Check sheet for the modelled part. Datum: model origin and axes. Units: mm. Face numbers are marked on the shaded views. Give positions to 0.01 mm unless a question says otherwise; leave off trailing zeros. Order: outer loops, then holes, each group sorted by start corner. A loop starts at its lowest first (then second) coordinate and runs counter-clockwise, first axis right, second up. Notation, with made-up numbers: (-1.5, 73) -> (2.5, 73) arc R15 cw to (2.5, 98) -> close; hole circle Ø10 at (80.25, 60.25). An arc over 180 degrees is marked (long way). Answer in a Markdown table with one row per item. Add a question column.
(1) Cross-section at D-D (y = 5). Record the cut outline in (x, z), then the cut area to 3 significant figures.
(2) Cross-section at A-A (z = 9.25). Record the cut outline in (x, y).
(3) Thickness scan on L1, parallel to Y at x = 15, z = 1.5; L2, parallel to X at y = 6, z = 7.75; L3, parallel to Y at x = -6.2, z = 13.25. Record the ranges inside material, lowest first. Write a range as [from, to].
(4) Release check for a two-part mould opening along X. For the marked faces 1, 2, 3 and 4 record: released by +X, released by -X, zero draft, split by the parting line, or undercut.
(5) Cross-section at C-C (z = 5.75). Record the cut outline in (x, y), then the cut area to 3 significant figures.
(6) Go/stop test with flat-tipped pins: pin 1 (1 mm diameter, centred on x = -11, y = 2, fed in from +Z); pin 2 (4.5 mm diameter, centred on y = -7.5, z = 5.75, fed in from +X); pin 3 (4.5 mm diameter, centred on y = 4, z = 10, fed in from -X); pin 4 (1.5 mm diameter, centred on x = 9, z = 5.5, fed in from -Y). Record where each tip stops, or that it passes through.
(7) Cross-section at B-B (x = 15). Record the cut outline in (y, z), then the cut area to 3 significant figures.
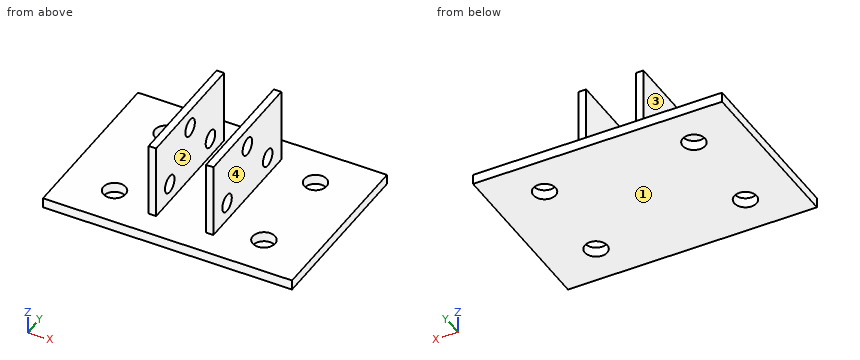
```python
from build123d import *

# Parameters (mm, degrees)
SKETCH2_W           = 50
SKETCH2_H           = 35
SKETCH2_R           = 2.25
BOSS_EXTRUDE1_DEPTH = 2
SKETCH3_W           = 1.5
SKETCH3_H           = 25
BOSS_EXTRUDE2_DEPTH = 15
SKETCH4_R           = 1.75
CUT_EXTRUDE1_DEPTH  = 32.5


with BuildPart() as part:
    # Sketch2 → Boss-Extrude1 (new body)
    with BuildSketch(Plane.XY):
        Rectangle(SKETCH2_W, SKETCH2_H)
        with Locations((15, 9.5)):
            Circle(SKETCH2_R, mode=Mode.SUBTRACT)
        with Locations((-15, 9.5)):
            Circle(SKETCH2_R, mode=Mode.SUBTRACT)
        with Locations((-15, -9.5)):
            Circle(SKETCH2_R, mode=Mode.SUBTRACT)
        with Locations((15, -9.5)):
            Circle(SKETCH2_R, mode=Mode.SUBTRACT)
    extrude(amount=BOSS_EXTRUDE1_DEPTH)

    # Sketch3 → Boss-Extrude2 (add)
    with BuildSketch(Plane.XY.offset(2)):
        with Locations((-5.75, 0)):
            Rectangle(SKETCH3_W, SKETCH3_H)
        with Locations((5.75, 0)):
            Rectangle(SKETCH3_W, SKETCH3_H)
    extrude(amount=BOSS_EXTRUDE2_DEPTH)

    # Sketch4 → Cut-Extrude1 (cut, through all)
    with BuildSketch(Plane.ZY.offset(6.5)):
        with Locations((5.75, -7.5)):
            Circle(SKETCH4_R)
        with Locations((5.75, 7.5)):
            Circle(SKETCH4_R)
        with Locations((13.25, 0)):
            Circle(SKETCH4_R)
    extrude(amount=-CUT_EXTRUDE1_DEPTH, mode=Mode.SUBTRACT)


solid = part.part
```
Answer below:
| question | item | result |
|---|---|---|
| 1 | outline | (-25, 0) -> (25, 0) -> (25, 2) -> (6.5, 2) -> (6.5, 17) -> (5, 17) -> (5, 2) -> (-5, 2) -> (-5, 17) -> (-6.5, 17) -> (-6.5, 2) -> (-25, 2) -> close |
| 1 | area | 145 mm² |
| 2 | outline | (-6.5, -12.5) -> (-5, -12.5) -> (-5, 12.5) -> (-6.5, 12.5) -> close; (5, -12.5) -> (6.5, -12.5) -> (6.5, 12.5) -> (5, 12.5) -> close |
| 3 | L1 | y = [-17.5, -11.75], [-7.25, 7.25], [11.75, 17.5] |
| 3 | L2 | x = [-6.5, -5], [5, 6.5] |
| 3 | L3 | y = [-12.5, -1.75], [1.75, 12.5] |
| 4 | face 1 | zero draft |
| 4 | face 2 | undercut |
| 4 | face 3 | released by -X |
| 4 | face 4 | released by +X |
| 5 | outline | (-6.5, -12.5) -> (-5, -12.5) -> (-5, -9.25) -> (-6.5, -9.25) -> close; (-6.5, -5.75) -> (-5, -5.75) -> (-5, 5.75) -> (-6.5, 5.75) -> close; (-6.5, 9.25) -> (-5, 9.25) -> (-5, 12.5) -> (-6.5, 12.5) -> close; (5, -12.5) -> (6.5, -12.5) -> (6.5, -9.25) -> (5, -9.25) -> close; (5, -5.75) -> (6.5, -5.75) -> (6.5, 5.75) -> (5, 5.75) -> close; (5, 9.25) -> (6.5, 9.25) -> (6.5, 12.5) -> (5, 12.5) -> close |
| 5 | area | 54.0 mm² |
| 6 | pin 1 | stops at z = 2 |
| 6 | pin 2 | stops at x = 6.5 |
| 6 | pin 3 | stops at x = -6.5 |
| 6 | pin 4 | passes through |
| 7 | outline | (-17.5, 0) -> (-11.75, 0) -> (-11.75, 2) -> (-17.5, 2) -> close; (-7.25, 0) -> (7.25, 0) -> (7.25, 2) -> (-7.25, 2) -> close; (11.75, 0) -> (17.5, 0) -> (17.5, 2) -> (11.75, 2) -> close |
| 7 | area | 52.0 mm² |
